Design review of the part shown in the three views and the two pictorial views. Dimensions are in mm from the part's minimum x, y and z. A direction names the side the tool comes from. Give positions to 0.01 mm unless a question says otherwise; leave off trailing zeros. Loops run counter-clockwise (first coordinate to the right, second up) from the corner with the lowest first, then second, coordinate; pieces in that order, holes last. Notation, with made-up numbers: (-27, -24) - (-17, -24) arc R14 ccw to (-17, -3) - close; hole circle Ø9 at (-25.75, -36). An arc over 180 degrees is marked (long way). Put each result on its own line as item: value. Start each with the question number.
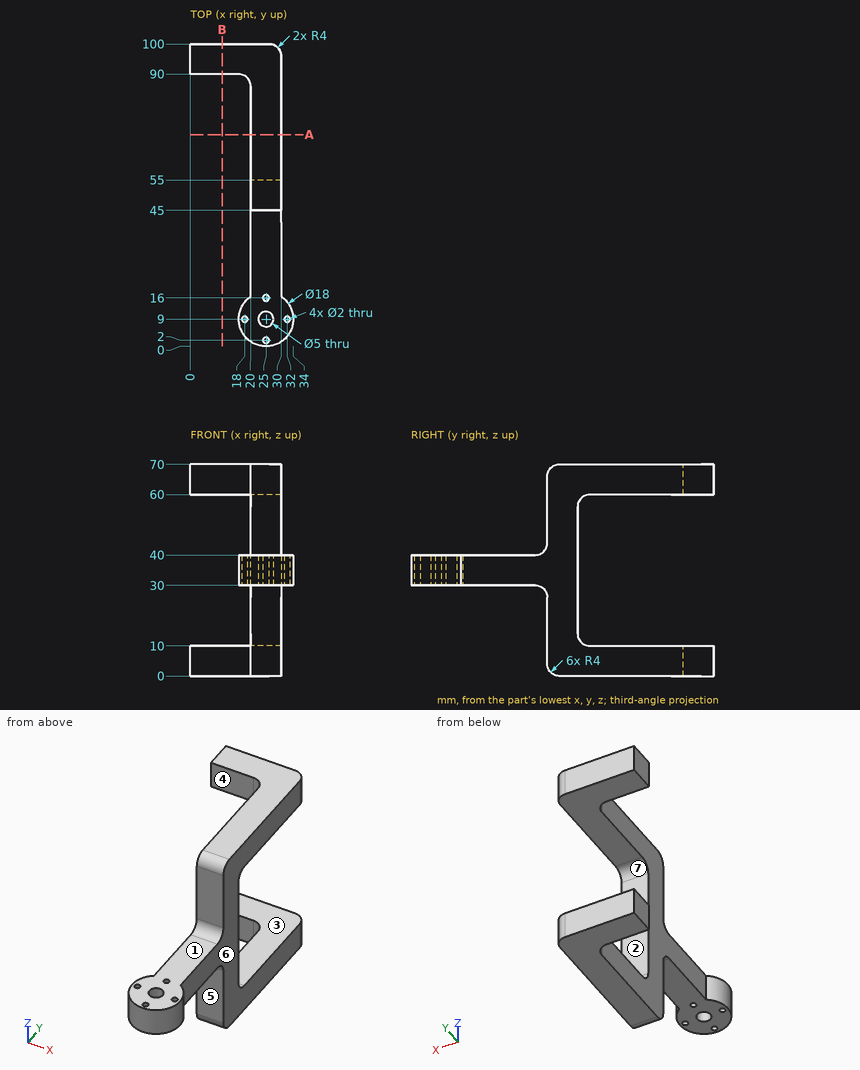
1) Mouldability with a two-part tool opening along Z and no side actions: class the marked faces 1, 2, 3 and 4 as released by +Z, released by -Z, zero draft, split by the parting line, or undercut.
2) Insertion check: P1, Ø11, axis at x = 27, z = 25, coming from the +Y side; P2, Ø8, axis at x = 11, z = 3, coming from the -Y side; P3, Ø1.8, axis at x = 18, y = 9, coming from the -Z side; P4, Ø5, axis at x = 26, y = 21, coming from the +Z side. Each pin has a flat end and moves straight along its axis. Give the tip position at first contact, or say it passes through.
3) Wall thickness on probe 1 along Y at (x, z) = (25, 33.5); probe 2 along Z at (x, y) = (11, 93); probe 3 along Y at (x, z) = (7, 3): over which ranges is each line inside the solid? List them lowest first.
4) Machinability: for the marked faces 5, 6 and 7, which of the approach directions +Z, -Z, +X, -X, +Y, -Y give a long, thin tool a straight path to every point of the face, cutting with its end or side? Answer none if there is none.
5) Take a section at A-A on y = 70. State the section outline as (x, z) points, and give its area (3 significant figures).
6) Take a section at B-B on x = 10.5. State the section outline as (y, z) points.
Answers follow:
1. face 1: released by +Z
1. face 2: undercut
1. face 3: undercut
1. face 4: zero draft
2. P1: y = 55
2. P2: y = 90
2. P3: through
2. P4: z = 40
3. probe 1: 0 to 1, 3 to 6.5, 11.5 to 15, 17 to 55
3. probe 2: 0 to 10, 60 to 70
3. probe 3: 90 to 100
4. face 5: -Z, +X, -X, -Y
4. face 6: +Z, -Z, +X, +Y
4. face 7: +X, -X, +Y
5. outline: (20, 0) - (30, 0) - (30, 10) - (20, 10) - close; (20, 60) - (30, 60) - (30, 70) - (20, 70) - close
5. area: 200 mm2
6. outline: (90, 0) - (100, 0) - (100, 10) - (90, 10) - close; (90, 60) - (100, 60) - (100, 70) - (90, 70) - close
